The figure shows three views and two pictorial views of one solid part (mm, origin at its lowest corner). Answer the questions. Round coordinates to 2 decimals unless told otherwise and drop trailing zeros. Loops run counter-clockwise (first coordinate to the right, second up) from the corner with the lowest first, then second, coordinate; pieces in that order, holes last. Notation, with made-up numbers: (-5, 86.25) -> (27, 86.25) arc R37 cw to (27, 123.25) -> close; hole circle Ø11 at (39.25, 8). An arc over 180 degrees is marked (long way). Use a Markdown table: item, result. Add a question column.
Q1. Section A-A on z = 8.5 is taken. Give the vertices of the cut face in (x, y), then the cut area to 3 significant figures.
Q2. Consider line 1 (X direction, y = 4.5, z = 6); line 2 (Y direction, x = 29, z = 18); line 3 (Y direction, x = 47, z = 6). Determine where each line is inside the solid, lowest interval first.
Q3. Given pin 1 Ø2 at (x, z) = (93.5, 30.5) entering from -Y; pin 2 Ø5 at (x, y) = (112.5, 12.5) entering from +Z; pin 3 Ø2 at (x, z) = (65, 7.5) entering from +Y, each flat-ended and moving along its own axis, determine where each tip first touches the part or whether it passes through.
Q4. Section C-C on x = 33 is taken. Give the vertices of the cut face in (y, z), then the cut area to 3 significant figures.
Q5. For a pull along X with two mould halves and no side action, classify the marked faces 1, 2 and 3 as released by +X, released by -X, zero draft, split by the parting line, or undercut.
Q6. Section B-B on y = 17.5 is taken. Give the vertices of the cut face in (x, z), then the cut area to 3 significant figures.
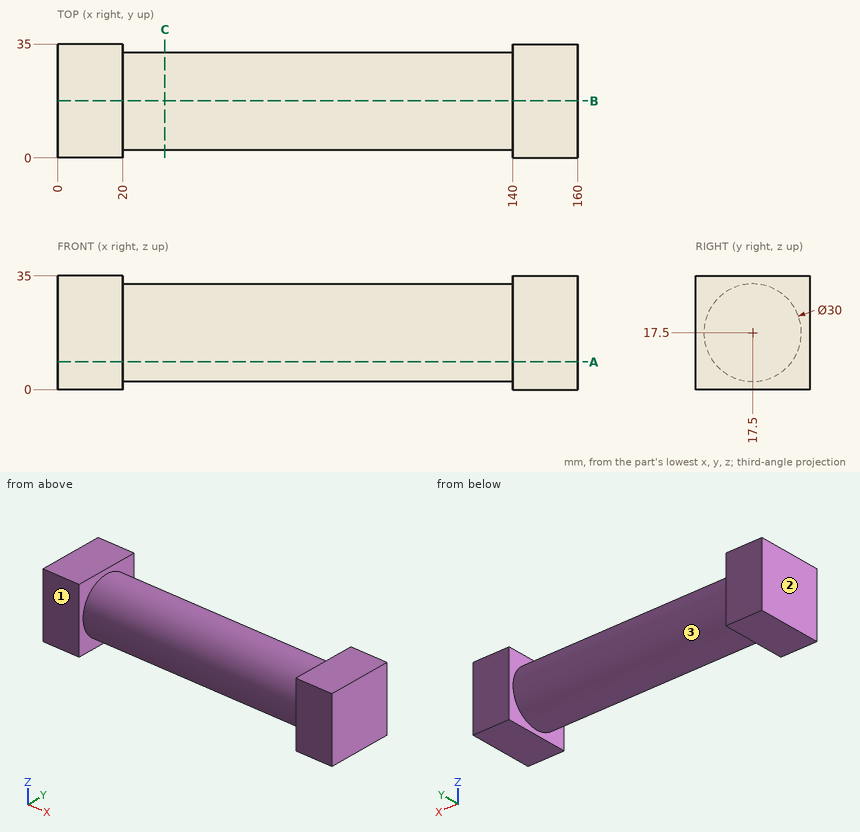
Checked values:
| question | item | result |
|---|---|---|
| 1 | outline | (0, 0) -> (20, 0) -> (20, 5.5) -> (140, 5.5) -> (140, 0) -> (160, 0) -> (160, 35) -> (140, 35) -> (140, 29.5) -> (20, 29.5) -> (20, 35) -> (0, 35) -> close |
| 1 | area | 4,280 mm2 |
| 2 | line 1 | x = 0 to 20, 140 to 160 |
| 2 | line 2 | y = 2.51 to 32.49 |
| 2 | line 3 | y = 7.87 to 27.13 |
| 3 | pin 1 | stops at y = 8.5 |
| 3 | pin 2 | stops at z = 32.29 |
| 3 | pin 3 | stops at y = 29.5 |
| 4 | outline | circle Ø30 at (17.5, 17.5) |
| 4 | area | 707 mm2 |
| 5 | face 1 | zero draft |
| 5 | face 2 | released by -X |
| 5 | face 3 | undercut |
| 6 | outline | (0, 0) -> (20, 0) -> (20, 2.5) -> (140, 2.5) -> (140, 0) -> (160, 0) -> (160, 35) -> (140, 35) -> (140, 32.5) -> (20, 32.5) -> (20, 35) -> (0, 35) -> close |
| 6 | area | 5,000 mm2 |
